Autodesk Inventor part; units mm, degrees
ref_plane "YZ Plane" through (0, 0, 0) normal (1, 0, 0) x (0, 1, 0)
ref_plane "XZ Plane" through (0, 0, 0) normal (0, 1, 0) x (-1, 0, 0)
ref_plane "XY Plane" through (0, 0, 0) normal (0, 0, 1) x (1, 0, 0)
sketch "Sketch1" plane through (0, 0, 0) normal (0, 0, 1) x (1, 0, 0)
  line L0 (8.7118, -48.8173) -> (8.7118, -78.8173)
  line L1 (5.5118, -78.8173) -> (8.7118, -78.8173)
  line L2 (5.5118, 131.1827) -> (5.5118, -108.8173)
  line L3 (5.5118, 131.1827) -> (5.5118, -141.2563)
  line L4 (5.5118, -141.2563) -> (25.5118, -161.2563)
  line L5 (25.5118, -161.2563) -> (40.5118, -161.2563)
  line L6 (14.7118, -45.3532) -> (8.7118, -48.8173)
  line L7 (14.7118, -35.3532) -> (14.7118, -45.3532)
  circle A0 centre (11.7118, -40.3532) radius 1.85
  line L8 (8.7118, -31.8891) -> (14.7118, -35.3532)
  line L9 (8.7118, -78.8173) -> (8.7118, -140.2136)
  line L10 (8.7118, -140.2136) -> (26.7544, -158.2563)
  line L11 (26.7544, -158.2563) -> (40.5118, -158.2563)
  line L12 (40.5118, -158.2563) -> (40.5118, -161.2563)
  point P0 (0, 0)
  point P1 (33.0118, -161.2563)
  dimension "d0" = 3
  dimension "d1" = 3
extrude "Extrusion1" add sketch "Sketch1" along normal blind 64 contours L1 L9 L10 L11 L12 L5 L4 L3 L2
sketch "Sketch2" plane through (0, 0, 64) normal (0, 0, 1) x (1, 0, 0)
  line L0 (8.7118, -140.2136) -> (8.7118, -78.8173)
  line L1 (26.7544, -158.2563) -> (8.7118, -140.2136)
  circle A0 centre (12.7118, -101.131) radius 1.75
  circle A1 centre (19.3686, -145.2136) radius 1.75
  line L2 (26.7544, -158.2563) -> (26.7544, -146.9426)
  line L3 (26.7544, -146.9426) -> (16.7118, -136.8999)
  line L4 (16.7118, -136.8999) -> (16.7118, -97.131)
  line L5 (16.7118, -97.131) -> (13.3981, -93.8173)
  line L6 (13.3981, -93.8173) -> (8.7118, -93.8173)
  line L7 (8.7118, -140.2136) -> (8.7118, -78.8173)
  point P0 (0, 0)
  dimension "d4" = 4
  dimension "d5" = 4
  dimension "d6" = 3.5
  dimension "d7" = 4
  dimension "d8" = 4
  dimension "d9" = 45
  dimension "d10" = 4
  dimension "d11" = 5
  dimension "d12" = 15
extrude "Extrusion2" add sketch "Sketch2" against normal blind 3
equation "\"d5\" = d4"
equation "\"d7\" = d5"
equation "\"d8\" = d7"
equation "\"d10\" = d4"
properties part number "Drag Chain Edge Panel" material "ABS Plastic"
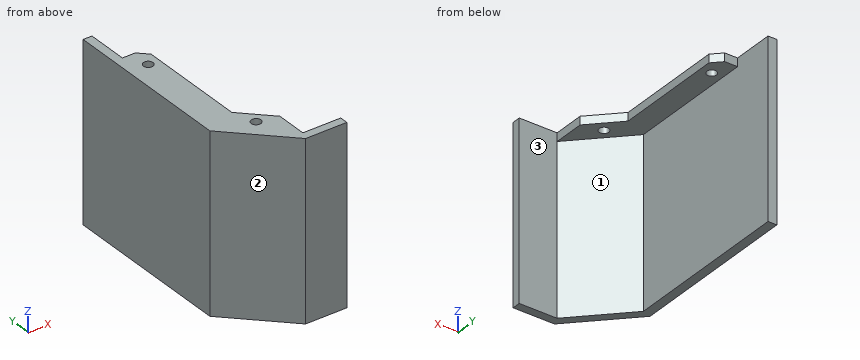
Part model, mm, in its own coordinate system. Face numbers are marked on the shaded views. A direction names the side the tool comes from. Round coordinates to 2 decimals unless told otherwise and drop trailing zeros. Write each loop counter-clockwise with the first axis right and the second up, starting at its lowest first coordinate (ties: lowest second). Pieces come first, ordered by that corner, then holes. Notation, with made-up numbers: M 22.25,4 L 34.25,4 A17 ccw 34.25,18 Z; hole C -13,-8 d6. An arc over 180 degrees is marked long. One line per question, with ' | ' between items.
(1) Saw through at B-B on x = 19. Write the cut outline in (y, z), then the cut area to 3 significant figures.
Answer key:
outline: M -154.74,0 L -150.5,0 L -150.5,61 L -146.92,61 L -146.92,64 L -154.74,64 Z; M -143.5,61 L -139.19,61 L -139.19,64 L -143.5,64 Z | area: 295 mm^2
(2) 3-axis set-ups, long thin cutter, end or side, ignore diameter. For the marked faces 1, 2 and 3: which of +Z, -Z, +X, -X, +Y, -Y reach the whole face in a straight line?
Answer key:
face 1: -Z, +X, +Y | face 2: +Z, -Z, -X, -Y | face 3: +Z, -Z, +X, +Y
(3) Saw through at D-D on x = 30.5. Write the cut outline in (y, z), then the cut area to 3 significant figures.
Answer key:
outline: M -161.26,0 L -158.26,0 L -158.26,64 L -161.26,64 Z | area: 192 mm^2
(4) Pin check, flat tips, straight feed: pin 1 (1.5 mm diameter, centred on y = -154.5, z = 62.5, fed in from +X); pin 2 (1.5 mm diameter, centred on y = -99, z = 23.5, fed in from +X); pin 3 (3.5 mm diameter, centred on x = 11.5, z = 62, fed in from +Y). Stop position of each tip, or through.
Answer key:
pin 1: stops at x = 26.75 | pin 2: stops at x = 8.71 | pin 3: stops at y = -93.82
(5) Probe line 1 along Z through (x, y) = (17, -138); line 2 along X through (y, z) = (-100, 52); line 3 along Y through (x, z) = (29, 39). List the from-to ranges inside material, lowest first.
Answer key:
line 1: z = 61 to 64 | line 2: x = 5.51 to 8.71 | line 3: y = -161.26 to -158.26
(6) Saw through at C-C on y = -118. Write the cut outline in (x, z), then the cut area to 3 significant figures.
Answer key:
outline: M 5.51,0 L 8.71,0 L 8.71,61 L 16.71,61 L 16.71,64 L 5.51,64 Z | area: 229 mm^2
(7) Saw through at A-A on z = 42.5. Write the cut outline in (x, y), then the cut area to 3 significant figures.
Answer key:
outline: M 5.51,-141.26 L 25.51,-161.26 L 40.51,-161.26 L 40.51,-158.26 L 26.75,-158.26 L 8.71,-140.21 L 8.71,-78.82 L 5.51,-78.82 Z | area: 322 mm^2
